Autodesk Fusion 360 part; units mm, degrees
sketch "Sketch1" plane through (0, 0, 0) normal (0, 0, 1) x (1, 0, 0)
  line L0 (-4.5, 12.5) -> (4.5, 12.5)
  line L1 (4.5, 12.5) -> (4.5, -12.5)
  line L2 (4.5, -12.5) -> (-4.5, -12.5)
  line L3 (-4.5, -12.5) -> (-4.5, 12.5)
  line L4 (-4.5, 12.5) -> (4.5, -12.5) construction
  line L5 (4.5, 12.5) -> (-4.5, -12.5) construction
  dimension "d1" = 9
  dimension "d2" = 25
extrude "Extrude1" add sketch "Sketch1" along normal blind 2
fillet "Fillet4" radius 2.5 4 edges at (4.5, 12.5, 1) (-4.5, 12.5, 1) (-4.5, -12.5, 1) (4.5, -12.5, 1)
sketch "Sketch7" plane through (0, 0, 2) normal (0, 0, 1) x (-1, 0, 0)
  arc A0 (-2, 12.5) -> (-4.5, 10) centre (-2, 10) ccw
  line L0 (-4.5, 10) -> (-4.5, -10)
  arc A1 (2, -12.5) -> (4.5, -10) centre (2, -10) ccw
  line L1 (4.5, -10) -> (4.5, 10)
  arc A2 (-4.5, -10) -> (-2, -12.5) centre (-2, -10) ccw
  line L2 (-2, -12.5) -> (2, -12.5)
  arc A3 (4.5, 10) -> (2, 12.5) centre (2, 10) ccw
  line L3 (2, 12.5) -> (-2, 12.5)
  line L4 (0, 12.5) -> (0, -12.5) construction
  line L5 (0, 12.5) -> (0, 8)
  line L6 (0, -12.5) -> (0, -8)
  circle A4 centre (0, -8) radius 1.2
  circle A5 centre (0, 8) radius 2.7
  dimension "d40" = 2.4
  dimension "d41" = 5.4
extrude "Extrude7" cut sketch "Sketch7" against normal blind 3 contours A4 | A5
Input: part model. Units: mm. Frame: model coordinates. Give positions to 0.01 mm unless a question says otherwise; leave off trailing zeros. Loops run counter-clockwise (first coordinate to the right, second up) from the corner with the lowest first, then second, coordinate; pieces in that order, holes last. Notation, with made-up numbers: M 46.25,35 L 70.25,35 A22 cw 70.25,73 Z; hole C 51,58.5 d11. An arc over 180 degrees is marked long. Use one line per item in the form item = value.
1. Line query: L1, parallel to Y at x = 0, z = 1.3; L2, parallel to X at y = 8, z = 0.9; L3, parallel to Y at x = -1, z = 1.5. Output: solid intervals per line, ascending.
Numbers:
L1 = -12.5 to -10.7, -5.3 to 6.8, 9.2 to 12.5
L2 = -4.5 to -1.2, 1.2 to 4.5
L3 = -12.5 to -10.51, -5.49 to 7.34, 8.66 to 12.5
2. Section query B-B, the plane y = -8. Return the cut outline in (x, z).
Numbers:
outline = M -4.5,0 L -2.7,0 L -2.7,2 L -4.5,2 Z; M 2.7,0 L 4.5,0 L 4.5,2 L 2.7,2 Z
3. Section query C-C, the plane z = 1.45. Return the cut outline in (x, y).
Numbers:
outline = M -4.5,-10 A2.5 ccw -2,-12.5 L 2,-12.5 A2.5 ccw 4.5,-10 L 4.5,10 A2.5 ccw 2,12.5 L -2,12.5 A2.5 ccw -4.5,10 Z; hole C 0,-8 d5.4; hole C 0,8 d2.4
4. Pull-direction query (Y, two-part tool) for faces 1 (the face through (-3.748, 11.787, 1.014)), 2 (the face through (-0.65, 6.99, 1.01)), 3 (the face through (4.5, 0, 1)); classes: released by +Y, released by -Y, zero draft, split by the parting line, or undercut.
Numbers:
face_1 = released by +Y
face_2 = undercut
face_3 = zero draft
5. Section query A-A, the plane x = 0. Return the cut outline in (y, z).
Numbers:
outline = M -12.5,0 L -10.7,0 L -10.7,2 L -12.5,2 Z; M -5.3,0 L 6.8,0 L 6.8,2 L -5.3,2 Z; M 9.2,0 L 12.5,0 L 12.5,2 L 9.2,2 Z
6. Section query D-D, the plane x = -2.25. Return the cut outline in (y, z), and give its area (3 significant figures).
Numbers:
outline = M -12.49,0 L -9.49,0 L -9.49,2 L -12.49,2 Z; M -6.51,0 L 12.49,0 L 12.49,2 L -6.51,2 Z
area = 44.0 mm²
